from build123d import *

# Parameters (mm, degrees)
SKETCH1_W            = 4
SKETCH1_H            = 14
BOSS_EXTRUDE1_DEPTH  = 3
SKETCH2_R            = 1.4
BOSS_EXTRUDE2_DEPTH  = 16
FILLET1_RADIUS       = 2
FILLET1_LENGTH       = 3
SKETCH3_W            = 4
SKETCH3_H            = 1
BOSS_EXTRUDE4_DEPTH  = 6
SKETCH6_R            = 1.6
CUT_EXTRUDE2_DEPTH   = 6
SKETCH7_W            = 3
SKETCH7_H            = 2
BOSS_EXTRUDE5_DEPTH  = 30.95
SKETCH8_W            = 3
SKETCH8_H            = 2
BOSS_EXTRUDE6_DEPTH  = 1
SKETCH9_W            = 1
SKETCH9_H            = 2
BOSS_EXTRUDE7_DEPTH  = 3
SKETCH10_W           = 1
SKETCH10_H           = 2
BOSS_EXTRUDE8_DEPTH  = 5.92
SKETCH11_W           = 1
SKETCH11_H           = 2
BOSS_EXTRUDE9_DEPTH  = 4
SKETCH12_W           = 1
SKETCH12_H           = 3
BOSS_EXTRUDE14_DEPTH = 0.93
SKETCH13_W           = 3
SKETCH13_H           = 3
BOSS_EXTRUDE15_DEPTH = 7.1


with BuildPart() as part:
    # Sketch1 → Boss-Extrude1 (new body)
    with BuildSketch(Plane.XY):
        with Locations((-1.434146341, -3.597560976)):
            Rectangle(SKETCH1_W, SKETCH1_H)
    extrude(amount=BOSS_EXTRUDE1_DEPTH)

    # Sketch2 → Boss-Extrude2 (add)
    with BuildSketch(Plane(origin=(0, 0, 0), x_dir=(-1, 0, 0), z_dir=(0, 0, -1))):
        with Locations(Location((1.434146341, 1.802439024, 0), (0, 0, 180))):
            Circle(SKETCH2_R)
    extrude(amount=BOSS_EXTRUDE2_DEPTH)

    # Fillet1: full round fillet: the end face becomes a half cylinder, R = half its width
    fillet1_face = Plane((-1.434146341, 3.402439024, 1.5), x_dir=(0, 0, 1), z_dir=(0, 1, 0))  # on the end face: x along it, z out of the body
    fillet1_slab = fillet1_face.offset(-FILLET1_RADIUS / 2) * Box(FILLET1_LENGTH, 2 * FILLET1_RADIUS, FILLET1_RADIUS, mode=Mode.PRIVATE)  # the body's end, R deep
    fillet1_round = Plane((-1.434146341, 1.402439024, 1.5), x_dir=(0, 1, 0), z_dir=(0, 0, 1)) * Cylinder(FILLET1_RADIUS, FILLET1_LENGTH, mode=Mode.PRIVATE)  # its axis R under the face
    add(fillet1_slab - fillet1_round, mode=Mode.SUBTRACT)

    # Sketch3 → Boss-Extrude4 (add)
    with BuildSketch(Plane.XY.offset(3)):
        with Locations((-1.434146341, -10.097560976)):
            Rectangle(SKETCH3_W, SKETCH3_H)
    extrude(amount=BOSS_EXTRUDE4_DEPTH)

    # Sketch6 → Cut-Extrude2 (cut)
    with BuildSketch(Plane(origin=(0, -9.597560976, 0), x_dir=(1, 0, 0), z_dir=(0, 1, 0))):
        with Locations(Location((-1.434146341, -6, 0), (0, 0, 270))):
            Circle(SKETCH6_R)
    extrude(amount=-CUT_EXTRUDE2_DEPTH, mode=Mode.SUBTRACT)

    # Sketch7 → Boss-Extrude5 (add)
    with BuildSketch(Plane.ZY.offset(3.434146341)):
        with Locations((1.5, -2.497560976)):
            Rectangle(SKETCH7_W, SKETCH7_H)
    extrude(amount=BOSS_EXTRUDE5_DEPTH)

    # Sketch8 → Boss-Extrude6 (add)
    with BuildSketch(Plane.ZY.offset(34.384146341)):
        with Locations((1.5, -2.497560976)):
            Rectangle(SKETCH8_W, SKETCH8_H)
    extrude(amount=BOSS_EXTRUDE6_DEPTH)

    # Sketch9 → Boss-Extrude7 (add)
    with BuildSketch(Plane(origin=(0, 0, 0), x_dir=(-1, 0, 0), z_dir=(0, 0, -1))):
        with Locations((34.884146341, -2.497560976)):
            Rectangle(SKETCH9_W, SKETCH9_H)
    extrude(amount=BOSS_EXTRUDE7_DEPTH)

    # Sketch10 → Boss-Extrude8 (add)
    with BuildSketch(Plane(origin=(0, 0, -3), x_dir=(-1, 0, 0), z_dir=(0, 0, -1))):
        with Locations((34.884146341, -2.497560976)):
            Rectangle(SKETCH10_W, SKETCH10_H)
    extrude(amount=BOSS_EXTRUDE8_DEPTH)

    # Sketch11 → Boss-Extrude9 (add)
    with BuildSketch(Plane(origin=(0, 0, -8.92), x_dir=(-1, 0, 0), z_dir=(0, 0, -1))):
        with Locations((34.884146341, -2.497560976)):
            Rectangle(SKETCH11_W, SKETCH11_H)
    extrude(amount=BOSS_EXTRUDE9_DEPTH)

    # Sketch12 → Boss-Extrude14 (add)
    with BuildSketch(Plane.XZ.offset(3.497560976)):
        with Locations((-34.884146341, -9.28)):
            Rectangle(SKETCH12_W, SKETCH12_H)
    extrude(amount=BOSS_EXTRUDE14_DEPTH)

    # Sketch13 → Boss-Extrude15 (add)
    with BuildSketch(Plane.XZ.offset(3.497560976)):
        with Locations((-33.884146341, 1.5)):
            Rectangle(SKETCH13_W, SKETCH13_H)
    extrude(amount=BOSS_EXTRUDE15_DEPTH)


solid = part.part
Part model, mm, in its own coordinate system. A direction names the side the tool comes from. Coordinates: 2 decimals unless noted, no trailing zeros. Order: outer loops, then holes, each group sorted by start corner. A loop starts at its lowest first (then second) coordinate and runs counter-clockwise, first axis right, second up.
(1) Slice it at B-B, the plane y = -8.75. Write the cut outline in (x, z), and give its area (3 significant figures).
Check sheet entries:
outline: (-35.38, 0) - (-32.38, 0) - (-32.38, 3) - (-35.38, 3) - close; (-3.43, 0) - (0.57, 0) - (0.57, 3) - (-3.43, 3) - close
area: 21.0 mm2
(2) Slice it at C-C, the plane z = 0.5. Write the cut outline in (x, y).
Check sheet entries:
outline: (-35.38, -10.6) - (-32.38, -10.6) - (-32.38, -3.5) - (-3.43, -3.5) - (-3.43, -10.6) - (0.57, -10.6) - (0.57, 1.4) arc R2 ccw to (-3.43, 1.4) - (-3.43, -1.5) - (-35.38, -1.5) - close
(3) Probe L1, parallel to X at y = -10.35, z = 6; L2, parallel to Z at x = -2.5, y = 1.75; L3, parallel to Z at x = -8, y = -2. List the from-to ranges inside material, lowest first.
Check sheet entries:
L1: x = -3.43 to -3.03, 0.17 to 0.57
L2: z = -16 to 3
L3: z = 0 to 3
(4) Slice it at A-A, the plane z = 6. Write the cut outline in (x, y), and give its area (3 significant figures).
Check sheet entries:
outline: (-3.43, -10.6) - (-3.03, -10.6) - (-3.03, -9.6) - (-3.43, -9.6) - close; (0.17, -10.6) - (0.57, -10.6) - (0.57, -9.6) - (0.17, -9.6) - close
area: 0.800 mm2
(5) Pin check, flat tips, straight feed: pin 1 Ø8 at (x, z) = (-17, 6) entering from +Y; pin 2 Ø2.5 at (x, z) = (-1.43, 6) entering from -Y; pin 3 Ø4 at (x, y) = (-10.5, -3) entering from -Z; pin 4 Ø0.7 at (x, y) = (-35, -4) entering from -Z. Stop position of each tip, or through.
Check sheet entries:
pin 1: stops at y = -1.5
pin 2: passes through
pin 3: stops at z = 0
pin 4: stops at z = -10.78
(6) Tool access for faces 1 (the face through (-2.833, 1.741, -7.888)), 2 (the face through (-35, -3.498, -12)), 3 (the face through (-32.384, -7, 1)), 4 (the face through (-34.384, -3, -6)), 5 (the face through (-3.434, 0, 1)): list every direction of +Z, -Z, +X, -X, +Y, -Y with a clear straight run to the whole face (end or side of a thin tool).
Check sheet entries:
face 1: -Z
face 2: -Z, +X, -X, -Y
face 3: +Z, -Z, -Y
face 4: -Z, +X, +Y, -Y
face 5: +Z, -Z, -X, +Y
(7) Slice it at D-D, the plane y = -3. Write the cut outline in (x, z), and give its area (3 significant figures).
Check sheet entries:
outline: (-35.38, -12.92) - (-34.38, -12.92) - (-34.38, 0) - (0.57, 0) - (0.57, 3) - (-35.38, 3) - close
area: 121 mm2
(8) Pull direction Z, two halves, no side cores. Call faces 6 (the face through (-35, -4, -7.78)), 7 (the face through (-2.047, -10.091, 7.478)), 8 (the face through (-1, -10, 9)), 9 (the face through (-35.384, -3, -3)): pulls with the +Z half, pulls with the -Z half, needs draft (parallel to the pull), parting line crosses it, or undercut.
Check sheet entries:
face 6: undercut
face 7: undercut
face 8: pulls with the +Z half
face 9: needs draft
